For this review, use the dimensioned drawing (mm, ordinates from the lowest corner) and the shaded views. A direction names the side the tool comes from. Coordinates: 2 decimals unless noted, no trailing zeros. Loops run counter-clockwise (first coordinate to the right, second up) from the corner with the lowest first, then second, coordinate; pieces in that order, holes last. Notation, with made-up numbers: M -13.75,11.25 L 17.25,11.25 A20 ccw 17.25,31.25 Z; hole C 34.25,4 d9. An arc over 180 degrees is marked long. One line per item, written item: value.
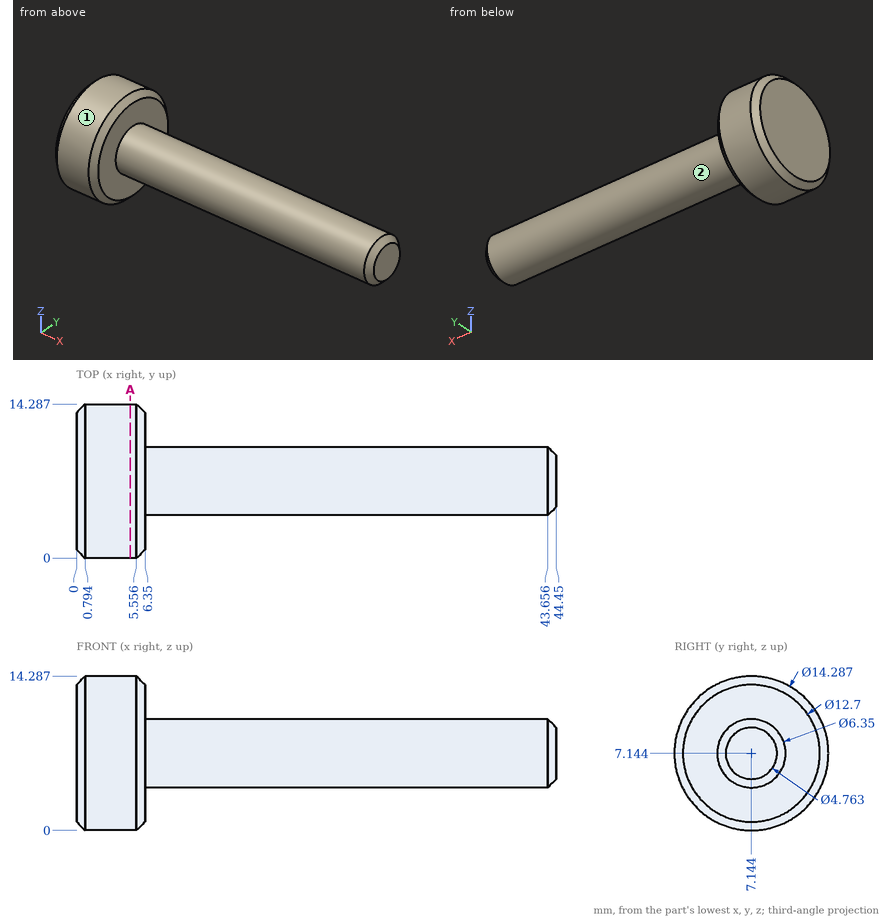
(1) To check wall thickness, follow line 1 along Z through (x, y) = (26, 7) (1 decimal); line 2 along X through (y, z) = (10.75, 11); line 3 along X through (y, z) = (13.75, 9) (1 decimal). State the ranges of each line that lie inside material, in increasing order. Write a range as [from, to].
Reply:
line 1: z = [4, 10.3]
line 2: x = [0, 6.35]
line 3: x = [0.5, 5.8]
(2) Tool access review of the marked faces 1 and 2: name each direction out of +Z, -Z, +X, -X, +Y, -Y from which nothing blocks a thin tool from reaching the whole face with its end or side.
Reply:
face 1: +X, -X
face 2: +X
(3) We need section A-A on x = 5. State the section outline as (y, z) points, then the cut area to 3 significant figures.
Reply:
outline: C 7.14,7.14 d14.29
area: 160 mm2
(4) Insertion check: pin 1 (1 mm diameter, centred on x = 21, z = 9, fed in from +Y) (1 decimal); pin 2 (6 mm diameter, centred on x = 19.5, y = 12.5, fed in from +Z); pin 3 (6 mm diameter, centred on x = 34.5, y = 6, fed in from +Z). Each pin has a flat end and moves straight along its axis. Give the tip position at first contact, or say it passes through.
Reply:
pin 1: stops at y = 10
pin 2: stops at z = 9.27
pin 3: stops at z = 10.32
